from build123d import *

# Parameters (mm, degrees)
F1_DEPTH = 10
F2_R     = 4.99999


# Not quite as in the source:
# - a fillet or chamfer is up to 0.001 mm smaller than in the source, because OpenCascade refuses the exact size


with BuildPart() as f1:
    # F0 (on Right) → F1 (new body)
    with BuildSketch(Plane.YZ):
        Polygon((0, 40), (0, 0), (150, 0), align=None)
        Polygon((2.5766265056, 49.662349396), (0, 40), (150, 0), (152.5766265056, 9.662349396), align=None)
    extrude(amount=F1_DEPTH)

    # F2 (radius 5 in the source; OpenCascade refuses exactly that, so slightly less here)
    f2_edges = [f1.edges().sort_by_distance(p)[0] for p in [
        (0, 77.576627, 29.662349),
        (10, 77.576627, 29.662349),
    ]]
    fillet(f2_edges, radius=F2_R)


solid = f1.part
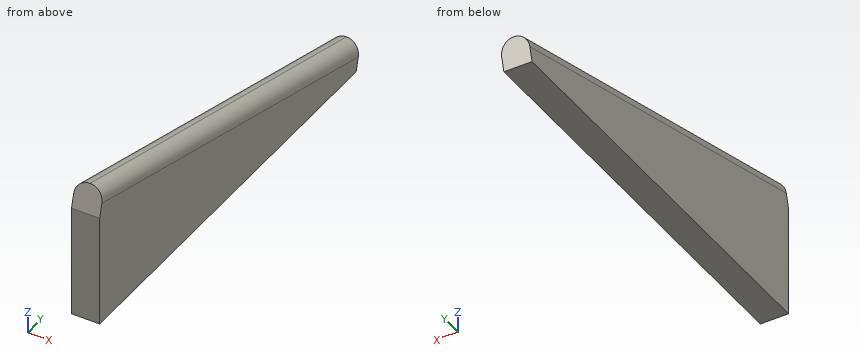
The listing builds one solid part. Answer for the finished solid, in the listing's coordinates (mm). Round coordinates to 2 decimals unless told otherwise and drop trailing zeros. Order: outer loops, then holes, each group sorted by start corner. A loop starts at its lowest first (then second) coordinate and runs counter-clockwise, first axis right, second up. Notation, with made-up numbers: M -28,-18.5 L -12,-18.5 A27 ccw -12,6.5 Z; hole C 50,-19 d3. An arc over 180 degrees is marked long. Answer in a Markdown table with one row per item. Add a question column.
1) The part is cut by section B-B on x = 2.5. Determine the outline of the cut face in (y, z), plus the area to 3 significant figures.
2) Flat-ended cylindrical pins translate along their axes: pin 1 Ø3 at (x, y) = (4, 69.5) entering from +Z; pin 2 Ø5 at (x, y) = (6.5, 100) entering from +Z. Find the tip coordinate at first contact, or state that the pin passes through.
3) Consider line 1 along Z through (x, y) = (9, 69); line 2 along Z through (x, y) = (4.5, 18); line 3 along Y through (x, z) = (2, 5.5). Determine where each line is inside the solid, lowest interval first. Write a range as from..to.
4) The part is cut by section A-A on x = 8.25. Determine the outline of the cut face in (y, z).
Findings below:
| question | item | result |
|---|---|---|
| 1 | outline | M 0,0 L 150,0 L 152.4,9.02 L 2.4,49.02 L 0,40 Z |
| 1 | area | 4,450 mm² |
| 2 | pin 1 | stops at z = 32.17 |
| 2 | pin 2 | stops at z = 24.27 |
| 3 | line 1 | z = 0..29.88 |
| 3 | line 2 | z = 0..45.52 |
| 3 | line 3 | y = 0..151.47 |
| 4 | outline | M 0,0 L 150,0 L 152.27,8.5 L 2.27,48.5 L 0,40 Z |
